from build123d import *

# Parameters (mm, degrees)
F0_R     = 32.5185756137
F1_DEPTH = 76.2
F2_R     = 5.08
F3_DEPTH = 124.714
F4_R     = 5.07999
F5_W     = 93.7804728746
F5_H     = 82.1867324412
F6_DEPTH = 14.732
F7_DEPTH = 36.83
F8_R     = 3.4460553294
F9_DEPTH = 19.558


# Not quite as in the source:
# - a fillet or chamfer is up to 0.001 mm smaller than in the source, because OpenCascade refuses the exact size


with BuildPart() as f1:
    # F0 (on Top) → F1 (new body)
    with BuildSketch(Plane.XY):
        Circle(F0_R)
    extrude(amount=F1_DEPTH)

    # F2
    f2_edges = [f1.edges().sort_by_distance(p)[0] for p in [
        (-32.518576, 0, 76.2),
    ]]
    fillet(f2_edges, radius=F2_R)

    # F3 (cut): a face of the model
    f3_faces = [f1.faces().sort_by_distance(p)[0] for p in [
        (0, 0, 76.2),
    ]]
    extrude(f3_faces, amount=-F3_DEPTH, mode=Mode.SUBTRACT)

    # F4 (radius 5.08 in the source; OpenCascade refuses exactly that, so slightly less here)
    f4_edges = [f1.edges().sort_by_distance(p)[0] for p in [
        (-32.518576, 0, 0),
    ]]
    fillet(f4_edges, radius=F4_R)

    # F5 (on Top) → F6 (join)
    with BuildSketch(Plane.XY):
        with Locations((0.0669173896, -1.1091846973)):
            Rectangle(F5_W, F5_H)
    extrude(amount=F6_DEPTH)

    # F7 (cut): a face of the model
    f7_faces = [f1.faces().sort_by_distance(p)[0] for p in [
        (0, 0, 14.732),
    ]]
    extrude(f7_faces, amount=-F7_DEPTH, mode=Mode.SUBTRACT)

    # F8 (on Top) → F9 (cut)
    with BuildSketch(Plane.XY):
        with Locations((-42.8946092725, 35.8311235905)):
            Circle(F8_R)
    extrude(amount=F9_DEPTH, mode=Mode.SUBTRACT)


solid = f1.part
Verification items for the finished model (mm, model axes). A direction names the side the tool comes from. Coordinates: 2 decimals unless noted, no trailing zeros. Write each loop counter-clockwise with the first axis right and the second up, starting at its lowest first coordinate (ties: lowest second). Pieces come first, ordered by that corner, then holes. Notation, with made-up numbers: M 23.5,88.25 L 54.5,88.25 A14 ccw 54.5,106.25 Z; hole C 17,47.25 d5. An arc over 180 degrees is marked long. Use a Markdown table: item, result.
Q1. Draft check along Y on faces 1 (the face through (-1, 39.984, 7)), 2 (the face through (-5.948, -26.786, 38.633)), 3 (the face through (-1, -42.203, 7)). Enter one of: +Y half, -Y half, draft (parallel to the pull), parting line (faces both ways), or undercut.
Reply:
| item | result |
|---|---|
| face 1 | +Y half |
| face 2 | undercut |
| face 3 | -Y half |
Q2. Sectioned sample at D-D, the plane x = -36.5. Record the boundary of the cut face in (y, z), plus the area to 3 significant figures.
Reply:
| item | result |
|---|---|
| outline | M -42.2,0 L 39.98,0 L 39.98,14.73 L -42.2,14.73 Z |
| area | 1,210 mm² |
Q3. Sectioned sample at A-A, the plane x = 0. Record the boundary of the cut face in (y, z), plus the area to 3 significant figures.
Reply:
| item | result |
|---|---|
| outline | M -42.2,0 L -27.44,0 L -27.44,76.2 A5.08 ccw -32.52,71.12 L -32.52,14.73 L -42.2,14.73 Z; M 27.44,0 L 39.98,0 L 39.98,14.73 L 32.52,14.73 L 32.52,71.12 A5.08 ccw 27.44,76.2 Z |
| area | 1,020 mm² |
Q4. Sectioned sample at C-C, the plane z = 17. Record the boundary of the cut face in (x, y), plus the area to 3 significant figures.
Reply:
| item | result |
|---|---|
| outline | C 0,0 d65.04; hole C 0,0 d54.88 |
| area | 957 mm² |
Q5. Sectioned sample at B-B, the plane y = 0. Record the boundary of the cut face in (x, z).
Reply:
| item | result |
|---|---|
| outline | M -46.82,0 L -27.44,0 L -27.44,76.2 A5.08 ccw -32.52,71.12 L -32.52,14.73 L -46.82,14.73 Z; M 27.44,0 L 46.96,0 L 46.96,14.73 L 32.52,14.73 L 32.52,71.12 A5.08 ccw 27.44,76.2 Z |
Q6. Thickness scan on line 1 (Y direction, x = 0, z = 47.5); line 2 (X direction, y = 1, z = 44.5); line 3 (Z direction, x = 33, y = 25). Record the ranges inside material, lowest first.
Reply:
| item | result |
|---|---|
| line 1 | y = -32.52 to -27.44, 27.44 to 32.52 |
| line 2 | x = -32.5 to -27.42, 27.42 to 32.5 |
| line 3 | z = 0 to 14.73 |
Q7. Set-up check for faces 4 (the face through (-32, -10, 14.732)), 5 (the face through (-43.34, 39.25, 7.26)): record each of +Z, -Z, +X, -X, +Y, -Y from which the full face is reachable in a straight line by a thin tool's end or side.
Reply:
| item | result |
|---|---|
| face 4 | +Z |
| face 5 | +Z, -Z |
Q8. Go/stop test with flat-tipped pins: P1, Ø5, axis at x = 31, y = 22.5, coming from the +Z side; P2, Ø10, axis at x = -18, z = 66.5, coming from the -Y side; P3, Ø12, axis at x = -25.5, y = 22, coming from the +Z side; P4, Ø5.5, axis at x = -42.89, y = 35.83, coming from the +Z side. Record where each tip stops, or that it passes through.
Reply:
| item | result |
|---|---|
| P1 | stops at z = 14.73 |
| P2 | stops at y = -29.81 |
| P3 | stops at z = 76.19 |
| P4 | passes through |
